Geometry: final body of the model. Coordinates: model frame, mm. Round coordinates to 2 decimals unless told otherwise and drop trailing zeros. Loops run counter-clockwise (first coordinate to the right, second up) from the corner with the lowest first, then second, coordinate; pieces in that order, holes last. Notation, with made-up numbers: M -9.75,-24.5 L 8.25,-24.5 A34 cw 8.25,11.5 Z; hole C 3,61 d8. An arc over 180 degrees is marked long. Write each question's results on one line, items separated by ' | '.
```python
from build123d import *

# Parameters (mm, degrees)
BOSS_EXTRUDE1_DEPTH = 2.921
BOSS_EXTRUDE2_DEPTH = 2.921


with BuildPart() as part:
    # Sketch1 → Boss-Extrude1 (new body)
    with BuildSketch(Plane(origin=(0, 0, 0), x_dir=(1, 0, 0), z_dir=(0, 1, 0))):
        Polygon((49.069031975, 13.148007491), (35.921024484, 35.921024484), (13.148007491, 49.069031975), (-13.148007491, 49.069031975), (-35.921024484, 35.921024484), (-49.069031975, 13.148007491), (-49.069031975, -13.148007491), (-35.921024484, -35.921024484), (-13.148007491, -49.069031975), (13.148007491, -49.069031975), (35.921024484, -35.921024484), (49.069031975, -13.148007491), align=None)
    extrude(amount=-BOSS_EXTRUDE1_DEPTH)

    # Sketch2 → Boss-Extrude2 (add)
    with BuildSketch(Plane(origin=(0, 0, 0), x_dir=(1, 0, 0), z_dir=(0, 1, 0))):
        Polygon((51.990031975, 13.930687082), (38.059344893, 38.059344893), (13.930687082, 51.990031975), (-13.930687082, 51.990031975), (-38.059344893, 38.059344893), (-51.990031975, 13.930687082), (-51.990031975, -13.930687082), (-38.059344893, -38.059344893), (-13.930687082, -51.990031975), (13.930687082, -51.990031975), (38.059344893, -38.059344893), (51.990031975, -13.930687082), align=None)
        Polygon((49.069031975, 13.148007491), (35.921024484, 35.921024484), (13.148007491, 49.069031975), (-13.148007491, 49.069031975), (-35.921024484, 35.921024484), (-49.069031975, 13.148007491), (-49.069031975, -13.148007491), (-35.921024484, -35.921024484), (-13.148007491, -49.069031975), (13.148007491, -49.069031975), (35.921024484, -35.921024484), (49.069031975, -13.148007491), align=None, mode=Mode.SUBTRACT)
    extrude(amount=-BOSS_EXTRUDE2_DEPTH)


solid = part.part
```
1. Section C-C (x = 41.5). Output: boundary loops of the cut face in (y, z), then the cut area to 3 significant figures.
Answer key:
outline: M -2.92,-32.1 L 0,-32.1 L 0,32.1 L -2.92,32.1 Z | area: 188 mm²
2. Section B-B (z = 43.5). Output: boundary loops of the cut face in (x, y), then the cut area to 3 significant figures.
Answer key:
outline: M -28.64,-2.92 L 28.64,-2.92 L 28.64,0 L -28.64,0 Z | area: 167 mm²
3. Section A-A (y = -1.55). Output: boundary loops of the cut face in (x, z), then the cut area to 3 significant figures.
Answer key:
outline: M -51.99,-13.93 L -38.06,-38.06 L -13.93,-51.99 L 13.93,-51.99 L 38.06,-38.06 L 51.99,-13.93 L 51.99,13.93 L 38.06,38.06 L 13.93,51.99 L -13.93,51.99 L -38.06,38.06 L -51.99,13.93 Z | area: 8,690 mm²
4. Ray query, probe 1 along X at (y, z) = (-1.35, 30.5); probe 2 along Z at (x, y) = (14, -2.4); probe 3 along Z at (x, y) = (18.5, -0.35). Return the intervals inside material, ascending.
Answer key:
probe 1: x = -42.42 to 42.42 | probe 2: z = -51.95 to 51.95 | probe 3: z = -49.35 to 49.35
5. Pin query (flat end, axial travel): P1, Ø1, axis at y = -2, z = 23, coming from the -X side. Return the tip coordinate at first contact, or that it passes through.
Answer key:
P1: stops at x = -47.04
